Input: dimensioned drawing with shaded views. Units: mm. Origin: part minimum x, y, z. A direction names the side the tool comes from. Round coordinates to 2 decimals unless told otherwise and drop trailing zeros. Write each loop counter-clockwise with the first axis right and the second up, starting at its lowest first coordinate (ties: lowest second). Pieces come first, ordered by that corner, then holes. Notation, with made-up numbers: M 88.5,69.25 L 130.5,69.25 A20 cw 130.5,103.25 Z; hole C 85,-39.75 d11. An arc over 180 degrees is marked long. Answer in a Markdown table with one row per item. Add a question column.
Item 1: Contact query for flat-ended pins moving along their axis: pin 1 (4 mm diameter, centred on x = 8, z = 2.5, fed in from -Y); pin 2 (1 mm diameter, centred on y = 8.5, z = 6.5, fed in from +X); pin 3 (10.5 mm diameter, centred on x = 15, y = 15, fed in from -Z); pin 4 (1.5 mm diameter, centred on x = 12, z = 8, fed in from +Y). Output: stop coordinate, or through.
Item 2: Material intervals for probe 1 along Y at (x, z) = (15, 11); probe 2 along Y at (x, z) = (15, 9.5); probe 3 along Z at (x, y) = (26, 7), sorted ascending.
Item 3: Cut plane C-C on x = 27. Return loops of the section in (y, z).
Item 4: Cut plane A-A on x = 15. Return loops of the section in (y, z), and give its area (3 significant figures).
Item 5: Set-up query: the marked faces 4, 5 and 6. Return all of +Z, -Z, +X, -X, +Y, -Y with unobstructed straight access to the full face (end or side cutting, diameter ignored); none if empty.
Item 6: Mould query, pull axis X, two halves, no side actions, for the marked faces 1, 2 and 3. Classes: released by +X, released by -X, zero draft, split by the parting line, or undercut.
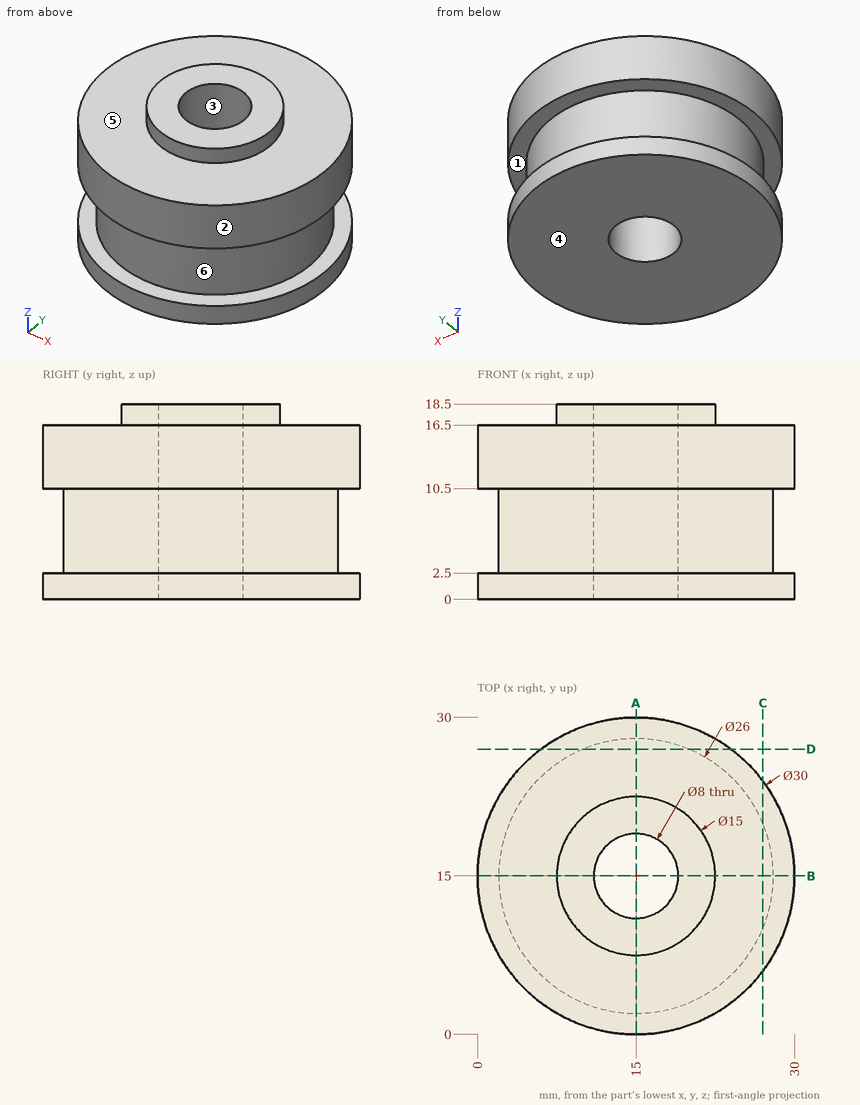
Results below:
| question | item | result |
|---|---|---|
| 1 | pin 1 | y = 0.86 |
| 1 | pin 2 | x = 26.53 |
| 1 | pin 3 | z = 0 |
| 1 | pin 4 | y = 27.8 |
| 2 | probe 1 | 0 to 11, 19 to 30 |
| 2 | probe 2 | 2 to 11, 19 to 28 |
| 2 | probe 3 | 0 to 2.5, 10.5 to 16.5 |
| 3 | outline | M 6,0 L 24,0 L 24,2.5 L 20,2.5 L 20,10.5 L 24,10.5 L 24,16.5 L 6,16.5 L 6,10.5 L 10,10.5 L 10,2.5 L 6,2.5 Z |
| 4 | outline | M 0,0 L 11,0 L 11,18.5 L 7.5,18.5 L 7.5,16.5 L 0,16.5 L 0,10.5 L 2,10.5 L 2,2.5 L 0,2.5 Z; M 19,0 L 30,0 L 30,2.5 L 28,2.5 L 28,10.5 L 30,10.5 L 30,16.5 L 22.5,16.5 L 22.5,18.5 L 19,18.5 Z |
| 4 | area | 345 mm2 |
| 5 | face 4 | -Z, +X, -X, +Y, -Y |
| 5 | face 5 | +Z |
| 5 | face 6 | none |
| 6 | face 1 | zero draft |
| 6 | face 2 | split by the parting line |
| 6 | face 3 | undercut |
